For this review, take the finished solid that the model builds, in its own axes (mm). Face numbers are marked on the shaded views. A direction names the side the tool comes from. Coordinates: 2 decimals unless noted, no trailing zeros. Loops run counter-clockwise (first coordinate to the right, second up) from the corner with the lowest first, then second, coordinate; pieces in that order, holes last. Notation, with made-up numbers: (62.5, 47.5) -> (118.5, 47.5) arc R12 cw to (118.5, 70.5) -> close; hole circle Ø3 at (49.5, 84.25). An arc over 180 degrees is marked (long way). Answer in a Markdown table with one row per item.
from build123d import *

# Parameters (mm, degrees)
F1_DEPTH  = 250
F3_DEPTH  = 238
F4_W      = 176
F4_H      = 43
F5_DEPTH  = 12.001
F6_R      = 10
F7_R      = 30
F8_R      = 20
F9_R      = 20
F10_DEPTH = 30


with BuildPart() as f1:
    # F0 (on Front) → F1 (new body)
    with BuildSketch(Plane.XZ):
        Polygon((200, 0), (98.472164, 1113.249898), (200, 1113.249898), (159.418754, 1550), (-159.418754, 1550), (-200, 1113.249898), (-98.472164, 1113.249898), (-200, 0), align=None)
        Polygon((-149.811608, 220), (-68.347662, 1113.249898), (68.347662, 1113.249898), (149.811608, 220), align=None, mode=Mode.SUBTRACT)
        Polygon((-167.083285, 1143.249898), (-132.077022, 1520), (132.077022, 1520), (167.083285, 1143.249898), align=None, mode=Mode.SUBTRACT)
    extrude(amount=F1_DEPTH)

    # F2 (on face) → F3 (cut)
    with BuildSketch(Plane(origin=(0, 0, 0), x_dir=(-1, 0, 0), z_dir=(0, 1, 0))):
        Polygon((152.547593, 190), (-152.547593, 190), (-167.139513, 30), (-87.5, 30), (-87.5, 38), (-60, 38), (-60, 30), (60, 30), (60, 38), (87.5, 38), (87.5, 30), (167.139513, 30), align=None)
    extrude(amount=-F3_DEPTH, mode=Mode.SUBTRACT)

    # F4 (on face) → F5 (cut, through all)
    with BuildSketch(Plane(origin=(0, -238, 0), x_dir=(-1, 0, 0), z_dir=(0, 1, 0))):
        with Locations((0, 59.5)):
            Rectangle(F4_W, F4_H)
    extrude(amount=-F5_DEPTH, mode=Mode.SUBTRACT)

    # F6
    f6_edges = [f1.edges().sort_by_distance(p)[0] for p in [
        (-149.811608, -125, 220),
        (149.811608, -125, 220),
        (-68.347662, -125, 1113.249898),
        (68.347662, -125, 1113.249898),
    ]]
    fillet(f6_edges, radius=F6_R)

    # F7
    f7_edges = [f1.edges().sort_by_distance(p)[0] for p in [
        (200, -125, 1113.249898),
        (-200, -125, 1113.249898),
        (-159.418754, -125, 1550),
        (159.418754, -125, 1550),
    ]]
    fillet(f7_edges, radius=F7_R)

    # F8
    f8_edges = [f1.edges().sort_by_distance(p)[0] for p in [
        (-167.083285, -125, 1143.249898),
        (-132.077022, -125, 1520),
        (132.077022, -125, 1520),
        (167.083285, -125, 1143.249898),
    ]]
    fillet(f8_edges, radius=F8_R)

    # F9 (on face) → F10 (cut, through all)
    with BuildSketch(Plane.XY.offset(1143.249898)):
        with Locations((0, -125)):
            Circle(F9_R)
    extrude(amount=-F10_DEPTH, mode=Mode.SUBTRACT)


solid = f1.part
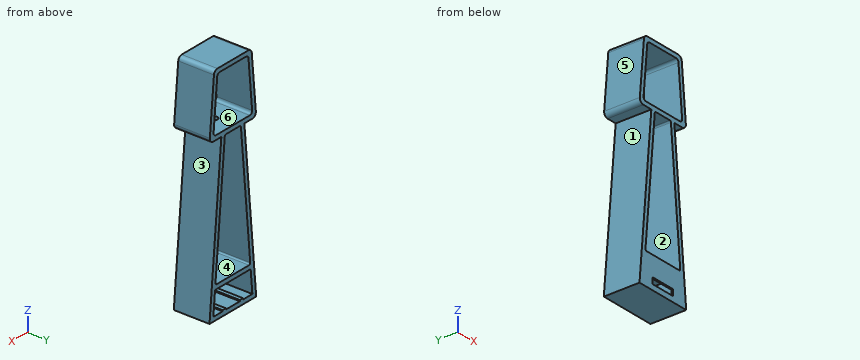
Item 1: For L1, parallel to Y at x = 0, z = 1129.25; L2, parallel to X at y = -131.5, z = 805; L3, parallel to X at y = -189, z = 430.5, list the stretches that pass through material, from the lowest coordinate up.
Worked answers:
| item | result |
|---|---|
| L1 | -250 to -145, -105 to 0 |
| L2 | -126.58 to -96.46, 96.46 to 126.58 |
| L3 | -160.74 to -130.61, 130.61 to 160.74 |
Item 2: The part is to be moulded in two halves that separate along X. For the marked faces 1, 2, 3 and 4, say which applies: +X half, -X half, draft (parallel to the pull), parting line (faces both ways), or undercut.
Worked answers:
| item | result |
|---|---|
| face 1 | -X half |
| face 2 | undercut |
| face 3 | +X half |
| face 4 | undercut |
Item 3: For the marked faces 5 and 6, list the 3-axis set-ups (+Z, -Z, +X, -X, +Y, -Y) from which the entire face can be reached by the end or side of a thin tool; tool diameter is ignored.
Worked answers:
| item | result |
|---|---|
| face 5 | +Z, -X, +Y, -Y |
| face 6 | +Y, -Y |
Item 4: Insertion check: pin 1 (10 mm diameter, centred on y = -164.5, z = 541.5, fed in from +X); pin 2 (5 mm diameter, centred on y = -122.5, z = 1357.5, fed in from -X); pin 3 (8 mm diameter, centred on y = -154, z = 975.5, fed in from -X). Each pin has a flat end and moves straight along its axis. Give the tip position at first contact, or say it passes through.
Worked answers:
| item | result |
|---|---|
| pin 1 | x = 151.07 |
| pin 2 | x = -177.54 |
| pin 3 | x = -111.4 |
Item 5: Take a section at C-C, the plane y = -125. Count the separate pieces of the cut face and the enclosed holes in it, and give its area (3 significant figures).
Worked answers:
| item | result |
|---|---|
| separate pieces | 1 |
| enclosed holes | 2 |
| area | 129,000 mm² |
Item 6: Take a section at A-A, the plane x = 0. State the section outline as (y, z) points.
Worked answers:
| item | result |
|---|---|
| outline | (-250, 0) -> (0, 0) -> (0, 30) -> (-238, 30) -> (-238, 38) -> (-250, 38) -> close; (-250, 81) -> (-238, 81) -> (-238, 190) -> (0, 190) -> (0, 220) -> (-250, 220) -> close; (-250, 1113.25) -> (-145, 1113.25) -> (-145, 1143.25) -> (-250, 1143.25) -> close; (-250, 1520) -> (0, 1520) -> (0, 1550) -> (-250, 1550) -> close; (-105, 1113.25) -> (0, 1113.25) -> (0, 1143.25) -> (-105, 1143.25) -> close |
Item 7: Take a section at D-D, the plane z = 161.5. State the section outline as (x, y) points, and give its area (3 significant figures).
Worked answers:
| item | result |
|---|---|
| outline | (-185.27, -250) -> (185.27, -250) -> (185.27, 0) -> (155.15, 0) -> (155.15, -238) -> (-155.15, -238) -> (-155.15, 0) -> (-185.27, 0) -> close |
| area | 18,800 mm² |
Item 8: Take a section at B-B, the plane z = 1207. State the section outline as (x, y) points.
Worked answers:
| item | result |
|---|---|
| outline | (-191.29, -250) -> (-161.16, -250) -> (-161.16, 0) -> (-191.29, 0) -> close; (161.16, -250) -> (191.29, -250) -> (191.29, 0) -> (161.16, 0) -> close |
